Autodesk Inventor part; units mm, degrees
ref_plane "YZ Plane" through (0, 0, 0) normal (1, 0, 0) x (0, 1, 0)
ref_plane "XZ Plane" through (0, 0, 0) normal (0, 1, 0) x (-1, 0, 0)
ref_plane "XY Plane" through (0, 0, 0) normal (0, 0, 1) x (1, 0, 0)
sketch "Sketch1" plane through (0, 0, 0) normal (0, 0, 1) x (1, 0, 0)
  line L0 (-17.5, 7.6319) -> (17.5, -9.8679)
  line L1 (17.5, -9.8679) -> (17.5, -7.6319)
  line L2 (17.5, -7.6319) -> (-17.5, 9.8679)
  line L3 (-17.5, 9.8679) -> (-17.5, 7.6319)
  line L4 (-7.5, -29.4219) -> (-3.6225, -29.4219)
  arc A0 (-1.9153, -30.38) -> (-3.6225, -29.4219) centre (-3.6225, -31.4219) ccw
  line L5 (-1.9153, -30.38) -> (2.2072, -37.135)
  arc A1 (2.5, -38.1769) -> (2.2072, -37.135) centre (0.5, -38.1769) ccw
  line L6 (2.5, -38.1769) -> (2.5, -47.4219)
  arc A2 (0.5, -49.4219) -> (2.5, -47.4219) centre (0.5, -47.4219) ccw
  line L7 (0.5, -49.4219) -> (-7.5, -49.4219)
  line L8 (-7.5, -49.4219) -> (-7.5, -29.4219)
  spline S0 degree 3 poles (6.0485, -14.3337) (6.0213, -14.5971) (5.9428, -14.8528) (5.6929, -15.3183) (5.524, -15.5241) (5.1467, -15.8339) (4.9505, -15.9462) (4.5292, -16.1007) (4.3073, -16.1418) (4.0832, -16.1449) knots 0 0 0 0 0.079442 0.079442 0.158531 0.158531 0.225919 0.225919 0.293184 0.293184 0.293184 0.293184
  line L9 (6.0485, -14.3337) -> (6.563, -9.3583)
  line L10 (6.563, -9.3583) -> (6.8849, -5.9915)
  arc A3 (6.8849, -5.9915) -> (5.7884, -4.0122) centre (4.894, -5.8011) ccw
  line L11 (-17.5, 7.6319) -> (5.7884, -4.0122)
  line L12 (-17.5, -57.5975) -> (-17.5, 7.6319)
  arc A4 (-4.376, -58.868) -> (-17.5, -57.5975) centre (-12.5, -74.368) ccw
  arc A5 (1.8324, -81.8643) -> (-4.376, -58.868) centre (-12.5, -73.3975) ccw
  line L13 (17.5, -78.3975) -> (17.5, -28.6365)
  ellipse E0 centre (15.5, -28.6365) end of major axis (15.5, -26.6191) minor radius 2 (17.5, -28.6365) -> (15.6888, -26.6281) ccw
  line L14 (15.6888, -26.6281) -> (3.1949, -25.4333)
  line L15 (3.1949, -25.4333) -> (4.0832, -16.1449)
  circle A6 centre (12, -52.3461) radius 1.25
  circle A7 centre (-5.3255, -52.3461) radius 1.25
  line L16 (14, -34.918) -> (10, -34.918)
  line L17 (14, -41.318) -> (14, -34.918)
  line L18 (10, -41.318) -> (14, -41.318)
  line L19 (10, -34.918) -> (10, -41.318)
  line L20 (-13.7851, -31.6782) -> (-9.7851, -31.6782)
  line L21 (-13.7851, -25.2782) -> (-13.7851, -31.6782)
  line L22 (-9.7851, -25.2782) -> (-13.7851, -25.2782)
  line L23 (-9.7851, -31.6782) -> (-9.7851, -25.2782)
  circle A8 centre (-7.1425, -17.0027) radius 1.25
  line L24 (-19.5, -83.5975) -> (-17.5, -83.5975)
  line L25 (-17.5, -57.5975) -> (-17.5, -83.5975)
  line L26 (-19.5, -57.5975) -> (-17.5, -57.5975)
  line L27 (-19.5, -57.5975) -> (-19.5, -83.5975)
  line L28 (-12.5, -83.5975) -> (-17.5, -83.5975)
  arc A9 (-12.5, -83.5975) -> (-6.9024, -81.9243) centre (-12.5, -73.3975) ccw
  line L29 (17.5, -7.6319) -> (18, -7.6319)
  line L30 (18, -7.6319) -> (18, -79.7438)
  line L31 (18, -79.7438) -> (17.5, -79.7438)
  line L32 (17.5, -79.7438) -> (17.5, -7.6319)
  line L33 (-6, -67.7722) -> (-6, -79.3975)
  line L34 (-12.5, -83.5975) -> (-17.5, -83.5975)
  arc A10 (-12.5, -83.5975) -> (-6.9024, -81.9243) centre (-12.5, -73.3975) ccw
  arc A11 (-6.9024, -81.9243) -> (-6, -80.2524) centre (-8, -80.2524) ccw
  line L35 (-6, -79.3975) -> (-6, -67.7722)
  line L36 (-6, -80.2524) -> (-6, -79.3975)
  line L37 (-19.5, -83.5975) -> (-6, -83.5975)
  line L38 (-6, -83.5975) -> (-6, -84.0975)
  line L39 (-6, -84.0975) -> (-19.5, -84.0975)
  line L40 (-19.5, -84.0975) -> (-19.5, -83.5975)
  line L41 (-6, -83.5975) -> (17.5, -78.3975)
  line L42 (16.4042, -78.64) -> (16.5122, -79.1281)
  line L43 (-3.7701, -83.1041) -> (-3.6621, -83.5922)
  line L44 (16.5122, -79.1281) -> (-3.6621, -83.5922)
  line L45 (16.5122, -79.1281) -> (21.5032, -78.0238)
  line L46 (-3.6621, -83.5922) -> (-17.5, -86.6542)
  line L47 (-6, -84.0975) -> (-5.7395, -84.0975)
  circle A12 centre (-12.5, -73.3975) radius 16.6465
  line L48 (1.8324, -81.8643) -> (17.5, -78.3975)
  point P0 (0, 0)
  point P1 (1.8324, -81.8643)
  point P2 (1.4649, -82.4578)
  point P3 (18, -78.7989)
  dimension "d0" = 0.5
  dimension "d1" = 0.5
  dimension "d4" = 0.5
  dimension "d5" = 0.5
extrude "Extrusion1" add sketch "Sketch1" against normal blind 100 contours L1 L29 L30 L45 L32 L13 | L32 L45 L42 L41 | L41 L42 L44 A12
ref_plane "Work Plane1" through (-19.5, -57.5975, -20) normal (0, 0, 1) x (1, 0, 0)
sketch "Sketch2" plane through (-19.5, -57.5975, -20) normal (0, 0, 1) x (1, 0, 0)
  line L0 (0, -26) -> (2, -26)
  line L1 (2, 0) -> (2, -26)
  line L2 (0, 0) -> (2, 0)
  line L3 (0, 0) -> (0, -26)
  line L4 (7, -26) -> (2, -26)
  arc A0 (7, -26) -> (12.5976, -24.3269) centre (7, -15.8) ccw
  line L5 (13.5, -21.8) -> (13.5, -10.1747)
  line L6 (0, -26) -> (13.5546, -26)
  line L7 (13.5546, -26) -> (13.5546, -26.5)
  line L8 (13.5546, -26.5) -> (0, -26.5)
  line L9 (0, -26.5) -> (0, -26)
  line L10 (37.5, -21.2015) -> (20.9649, -24.8603)
  line L11 (13.5546, -26.5) -> (20.9649, -24.8603)
  line L12 (20.9649, -24.8603) -> (37.5, -21.2015)
  line L13 (37.5, -21.2015) -> (37.5, 49.9656)
  line L14 (37.5, 49.9656) -> (37, 49.9656)
  line L15 (37, 49.9656) -> (37, -20.8)
  line L16 (37, -20.8) -> (21.3324, -24.2669)
  arc A1 (20.9649, -24.8603) -> (21.3324, -24.2669) centre (7, -15.8) ccw
  arc A2 (20.9649, -24.8603) -> (21.3324, -24.2669) centre (7, -15.8) ccw
  line L17 (21.3324, -24.2669) -> (13.5, -26)
  point P0 (19.5, 57.5975)
  dimension "d8" = 0.5
extrude "Extrusion2" add sketch "Sketch2" against normal blind 60 contours L0 L4 L6 L7 L8 L9 | L7 L6 L17 A1 L11
sketch "Sketch3" plane through (-19.5, -57.5975, -20) normal (0, 0, 1) x (1, 0, 0)
  line L0 (0, -26.5) -> (13.5546, -26.5)
  line L1 (13.5546, -26.5) -> (20.9649, -24.8603)
  arc A0 (20.9649, -24.8603) -> (21.3324, -24.2669) centre (7, -15.8) ccw
  line L2 (21.3324, -24.2669) -> (13.5, -26)
  line L3 (13.5, -26) -> (0, -26)
  line L4 (0, -26) -> (0, -26.5)
  point P0 (19.5, 57.5975)
  dimension "d11" = 167.523
properties part number "pokrywa" material "Aluminum 6061"
Build history of the part. All positions in model axes, mm. A direction names the side the tool comes from. Round coordinates to 2 decimals unless told otherwise and drop trailing zeros. Write each loop counter-clockwise with the first axis right and the second up, starting at its lowest first coordinate (ties: lowest second). Pieces come first, ordered by that corner, then holes. Notation, with made-up numbers: (22, -4) - (69, -4) arc R32 cw to (69, 29) - close; hole circle Ø10 at (-20, 7). An arc over 180 degrees is marked (long way). One line per question, with ' | ' between items.
1. Drop flat-ended pins along their axis: pin 1 Ø5 at (x, z) = (-8, -38.5) entering from +Y; pin 2 Ø2 at (y, z) = (-64, -64) entering from -X; pin 3 Ø0.7 at (x, y) = (-9, -83.5) entering from -Z; pin 4 Ø1.1 at (x, y) = (-10, -83) entering from +Z. Give the stop position or say it passes through.
Results are:
pin 1: y = -83.49 | pin 2: x = 17.5 | pin 3: z = -80 | pin 4: through
2. Band-saw the part on C-C, the plane x = 3.5. Write the cut outline in (y, z).
Results are:
outline: (-82.01, -100) - (-81.5, -100) - (-81.5, 0) - (-82.01, 0) - close
3. Band-saw the part on B-B, the plane y = -38.5. Write the cut outline in (x, z).
Results are:
outline: (17.5, -100) - (18, -100) - (18, 0) - (17.5, 0) - close
4. Tool access for faces 1 (the face through (-13, -83.598, -50)), 2 (the face through (-13, -84.098, -50)): list every direction of +Z, -Z, +X, -X, +Y, -Y with a clear straight run to the whole face (end or side of a thin tool).
Results are:
face 1: +Z, -Z, -X, +Y | face 2: +Z, -Z, +X, -X, -Y
5. Drill centre lines: line 1 along X through (y, z) = (-34, -19); line 2 along Y through (x, z) = (-15, -23); line 3 along Y through (x, z) = (16, -87.5). Where is each one in solid material? Low to high. Write a range as from..to.
Results are:
line 1: 17.5..18 | line 2: -84.1..-83.6 | line 3: -79.24..-78.73
6. Band-saw the part on A-A, the plane z = -88.5. Write the cut outline in (x, y), and give its area (3 significant figures).
Results are:
outline: (1.46, -82.46) - (16.51, -79.13) - (18, -78.8) - (18, -7.63) - (17.5, -7.63) - (17.5, -78.4) - (1.83, -81.86) arc R16.65 cw to start | area: 43.7 mm^2
